```python
from build123d import *
from build123d import SkipClean  # not in build123d's __all__

# Parameters (mm, degrees)
F1_DEPTH     = 2.5
F2_R         = 12
F2_R_2       = 9
F3_DEPTH     = 1.5
F5_DEPTH     = 3
F6_SIZE      = 1.99999
F7_SIZE      = 0.49999
F8_T3_ANGLE  = 65.5786890643
F8_T6_ANGLE  = 65.5786890643
F8_T9_ANGLE  = 65.5786890643
F8_T12_ANGLE = 65.5786890643


# Not quite as in the source:
# - a fillet or chamfer that OpenCascade refuses, or shapes differently, is made with other operations: its cross-section is extruded or revolved along the edge and cut away or added
# - a fillet or chamfer is up to 0.001 mm smaller than in the source, because OpenCascade refuses the exact size


with BuildPart() as f1:
    # F0 (on Front) → F1 (new body)
    with BuildSketch(Plane.XZ):
        with BuildLine():
            Line((-8.0321912081, 4.060037487), (-9.3329510623, 4.811031539))
            ThreePointArc((-9.3329510623, 4.811031539), (-10.5, 0), (-9.3329510623, -4.811031539))
            Line((-9.3329510623, -4.811031539), (-8.0321912081, -4.060037487))
            ThreePointArc((-8.0321912081, -4.060037487), (-9, 0), (-8.0321912081, 4.060037487))
        make_face()
    extrude(amount=-F1_DEPTH)



with BuildPart() as f1b:
    # F0 (on Front) → F1, piece 2 (new body)
    with BuildSketch(Plane.XZ):
        with BuildLine():
            ThreePointArc((8.8329510623, 5.6770569427), (0, 10.5), (-8.8329510623, 5.6770569427))
            Line((-8.8329510623, 5.6770569427), (-7.5321912081, 4.9260628908))
            ThreePointArc((-7.5321912081, 4.9260628908), (0, 9), (7.5321912081, 4.9260628908))
            Line((7.5321912081, 4.9260628908), (8.8329510623, 5.6770569427))
        make_face()
    extrude(amount=-F1_DEPTH)


with BuildPart() as f1c:
    # F0 (on Front) → F1, piece 3 (new body)
    with BuildSketch(Plane.XZ):
        with BuildLine():
            Line((8.0321912081, -4.060037487), (9.3329510623, -4.811031539))
            ThreePointArc((9.3329510623, -4.811031539), (10.5, 0), (9.3329510623, 4.811031539))
            Line((9.3329510623, 4.811031539), (8.0321912081, 4.060037487))
            ThreePointArc((8.0321912081, 4.060037487), (9, 0), (8.0321912081, -4.060037487))
        make_face()
    extrude(amount=-F1_DEPTH)


with BuildPart() as f1d:
    # F0 (on Front) → F1, piece 4 (new body)
    with BuildSketch(Plane.XZ):
        with BuildLine():
            Line((-7.5321912081, -4.9260628908), (-8.8329510623, -5.6770569427))
            ThreePointArc((-8.8329510623, -5.6770569427), (0, -10.5), (8.8329510623, -5.6770569427))
            Line((8.8329510623, -5.6770569427), (7.5321912081, -4.9260628908))
            ThreePointArc((7.5321912081, -4.9260628908), (0, -9), (-7.5321912081, -4.9260628908))
        make_face()
    extrude(amount=-F1_DEPTH)


with BuildPart() as f1_1:
    add(f1.part, clean=False)

    add(f1b.part)  # F3 merges F1b

    add(f1c.part)  # F3 merges F1c

    add(f1d.part)  # F3 merges F1d
    # F2 (on face) → F3 (join)
    with BuildSketch(Plane(origin=(0, 2.5, 0), x_dir=(-1, 0, 0), z_dir=(0, 1, 0))):
        Circle(F2_R)
        Circle(F2_R_2, mode=Mode.SUBTRACT)
    extrude(amount=F3_DEPTH)

    # F4 (on face) → F5 (join)
    with BuildSketch(Plane.XZ):
        with BuildLine():
            ThreePointArc((-7.5321912081, 4.9260628908), (0, 9), (7.5321912081, 4.9260628908))
            Line((7.5321912081, 4.9260628908), (8.8329510623, 5.6770569427))
            ThreePointArc((8.8329510623, 5.6770569427), (0, 10.5), (-8.8329510623, 5.6770569427))
            Line((-8.8329510623, 5.6770569427), (-7.5321912081, 4.9260628908))
        make_face()
        with BuildLine():
            Line((8.0321912081, -4.060037487), (9.7664331553, -5.0613025421))
            ThreePointArc((9.7664331553, -5.0613025421), (11, 0), (9.7664331553, 5.0613025421))
            Line((9.7664331553, 5.0613025421), (8.0321912081, 4.060037487))
            ThreePointArc((8.0321912081, 4.060037487), (9, 0), (8.0321912081, -4.060037487))
        make_face()
        with BuildLine():
            Line((-8.0321912081, 4.060037487), (-9.7664331553, 5.0613025421))
            ThreePointArc((-9.7664331553, 5.0613025421), (-11, 0), (-9.7664331553, -5.0613025421))
            Line((-9.7664331553, -5.0613025421), (-8.0321912081, -4.060037487))
            ThreePointArc((-8.0321912081, -4.060037487), (-9, 0), (-8.0321912081, 4.060037487))
        make_face()
        with BuildLine():
            Line((-7.5321912081, -4.9260628908), (-8.8329510623, -5.6770569427))
            ThreePointArc((-8.8329510623, -5.6770569427), (0, -10.5), (8.8329510623, -5.6770569427))
            Line((8.8329510623, -5.6770569427), (7.5321912081, -4.9260628908))
            ThreePointArc((7.5321912081, -4.9260628908), (0, -9), (-7.5321912081, -4.9260628908))
        make_face()
    with SkipClean():  # cleaning this boolean's faces spoils the solid; the shape is the same uncleaned
        extrude(amount=F5_DEPTH)

    # F6 (size 2 in the source; OpenCascade refuses exactly that, so slightly less here)
    f6_edges = [f1_1.edges().sort_by_distance(p)[0] for p in [
        (-11, -3, 0),
        (11, -3, 0),
    ]]
    chamfer(f6_edges, length=F6_SIZE)

    # F7 (size 0.5 in the source; OpenCascade refuses exactly that, so slightly less here)
    f7_edges = [f1_1.edges().sort_by_distance(p)[0] for p in [
        (-11, 0, 0),
        (11, 0, 0),
    ]]
    chamfer(f7_edges, length=F7_SIZE)

    # F8: fillet of radius 1 on 4 edges, made by hand


with BuildPart() as f8_tool1:
    # F8_s2 → F8_t3 (revolve)
    with BuildSketch(Plane(origin=(0, 0, 0), x_dir=(0, 1, 0), z_dir=(0.5415518782, 0, 0.8406673321))):
        with BuildLine():
            ThreePointArc((-0.5857964376, 11), (-0.96847987, 10.9238795325), (-1.2929032188, 10.7071067812))
            Line((-1.2929032188, 10.7071067812), (-1.00001, 11))
            Line((-1.00001, 11), (-0.5857964376, 11))
        make_face()
    revolve(axis=Axis((0, -1.00001, 0), (0, -1, 0)), revolution_arc=F8_T3_ANGLE)


with BuildPart() as f8_tool4:
    # F8_s5 → F8_t6 (revolve)
    with BuildSketch(Plane(origin=(0, 0, 0), x_dir=(0, 1, 0), z_dir=(0.5415518782, 0, 0.8406673321))):
        with BuildLine():
            ThreePointArc((-0.9142035624, 11), (-0.53152013, 10.9238795325), (-0.2070967812, 10.7071067812))
            Line((-0.2070967812, 10.7071067812), (-0.49999, 11))
            Line((-0.49999, 11), (-0.9142035624, 11))
        make_face()
    revolve(axis=Axis((0, -0.49999, 0), (0, -1, 0)), revolution_arc=F8_T6_ANGLE)


with BuildPart() as f8_tool7:
    # F8_s8 → F8_t9 (revolve)
    with BuildSketch(Plane(origin=(0, 0, 0), x_dir=(0, 1, 0), z_dir=(-0.5415518782, 0, -0.8406673321))):
        with BuildLine():
            ThreePointArc((-0.5857964376, 11), (-0.96847987, 10.9238795325), (-1.2929032188, 10.7071067812))
            Line((-1.2929032188, 10.7071067812), (-1.00001, 11))
            Line((-1.00001, 11), (-0.5857964376, 11))
        make_face()
    revolve(axis=Axis((0, -1.00001, 0), (0, -1, 0)), revolution_arc=F8_T9_ANGLE)


with BuildPart() as f8_tool10:
    # F8_s11 → F8_t12 (revolve)
    with BuildSketch(Plane(origin=(0, 0, 0), x_dir=(0, 1, 0), z_dir=(-0.5415518782, 0, -0.8406673321))):
        with BuildLine():
            ThreePointArc((-0.9142035624, 11), (-0.53152013, 10.9238795325), (-0.2070967812, 10.7071067812))
            Line((-0.2070967812, 10.7071067812), (-0.49999, 11))
            Line((-0.49999, 11), (-0.9142035624, 11))
        make_face()
    revolve(axis=Axis((0, -0.49999, 0), (0, -1, 0)), revolution_arc=F8_T12_ANGLE)


with BuildPart() as f1_2:
    add(f1_1.part, clean=False)

    # F8_t13: cut F8_tool1, F8_tool4, F8_tool7, F8_tool10
    add([f8_tool1.part, f8_tool4.part, f8_tool7.part, f8_tool10.part], mode=Mode.SUBTRACT)


solid = f1_2.part
```
Geometry check sheet. Reference: the model listing, model coordinates, mm. A direction names the side the tool comes from. Give positions to 0.01 mm unless a question says otherwise; leave off trailing zeros. Write each loop counter-clockwise with the first axis right and the second up, starting at its lowest first coordinate (ties: lowest second). Pieces come first, ordered by that corner, then holes. Notation, with made-up numbers: (77, -0.5) - (106, -0.5) arc R19 cw to (106, 6.5) - close; hole circle Ø9 at (-32, 66). An arc over 180 degrees is marked (long way). Use a Markdown table: item, result.
Q1. Section check B-B, the plane z = -7.25. Enter the section's corners in (x, y).
Computed:
| item | result |
|---|---|
| outline | (-9.56, 2.5) - (-7.6, 2.5) - (-7.6, -3) - (-5.33, -3) - (-5.33, 4) - (-9.56, 4) - close; (5.33, -3) - (7.6, -3) - (7.6, 2.5) - (9.56, 2.5) - (9.56, 4) - (5.33, 4) - close |
Q2. Thickness scan on L1, parallel to Z at x = 0, y = 0; L2, parallel to X at y = 2.75, z = 3.75; L3, parallel to Y at x = 7, z = -9.5. Record the ranges inside material, lowest first. Write a range as [from, to].
Computed:
| item | result |
|---|---|
| L1 | z = [-10.5, -9], [9, 10.5] |
| L2 | x = [-11.4, -8.18], [8.18, 11.4] |
| L3 | y = [2.5, 4] |
Q3. Draft check along Z on faces 4 (the face through (11.99, 3.24, 0.53)), 5 (the face through (0.1, -0.3, 10.5)), 6 (the face through (-8.173, -0.288, -5.296)). Enter one of: pulls with the +Z half, pulls with the -Z half, needs draft (parallel to the pull), parting line crosses it, or undercut.
Computed:
| item | result |
|---|---|
| face 4 | parting line crosses it |
| face 5 | pulls with the +Z half |
| face 6 | undercut |
Q4. Section check A-A, the plane y = 1.5. Enter the section's corners in (x, z).
Computed:
| item | result |
|---|---|
| outline | (-9.33, -4.81) - (-8.03, -4.06) arc R9 cw to (-8.03, 4.06) - (-9.33, 4.81) arc R10.5 ccw to start; (-8.83, -5.68) arc R10.5 ccw to (8.83, -5.68) - (7.53, -4.93) arc R9 cw to (-7.53, -4.93) - close; (-8.83, 5.68) - (-7.53, 4.93) arc R9 cw to (7.53, 4.93) - (8.83, 5.68) arc R10.5 ccw to start; (8.03, -4.06) - (9.33, -4.81) arc R10.5 ccw to (9.33, 4.81) - (8.03, 4.06) arc R9 cw to start |
Q5. Section check D-D, the plane y = -2. Enter the section's corners in (x, z).
Computed:
| item | result |
|---|---|
| outline | (-8.9, -4.56) - (-8.03, -4.06) arc R9 cw to (-8.03, 4.06) - (-8.9, 4.56) arc R10 ccw to start; (-8.83, -5.68) arc R10.5 ccw to (8.83, -5.68) - (7.53, -4.93) arc R9 cw to (-7.53, -4.93) - close; (-8.83, 5.68) - (-7.53, 4.93) arc R9 cw to (7.53, 4.93) - (8.83, 5.68) arc R10.5 ccw to start; (8.03, -4.06) - (8.9, -4.56) arc R10 ccw to (8.9, 4.56) - (8.03, 4.06) arc R9 cw to start |
Q6. Go/stop test with flat-tipped pins: P1, Ø4, axis at y = 1.5, z = 8, coming from the +X side; P2, Ø3, axis at x = -6.5, z = 5.5, coming from the +Y side; P3, Ø1.5, axis at x = -3, y = 2.5, coming from the +Z side. Record where each tip stops, or that it passes through.
Computed:
| item | result |
|---|---|
| P1 | stops at x = 10.23 |
| P2 | stops at y = 4 |
| P3 | stops at z = 11.79 |
Q7. Set-up check for faces 1 (the face through (-0.1, -0.3, -10.5)), 2 (the face through (10.5, 1.2, -0.1)), 3 (the face through (-10.5, 1.2, 0.1)): record each of +Z, -Z, +X, -X, +Y, -Y from which the full face is reachable in a straight line by a thin tool's end or side.
Computed:
| item | result |
|---|---|
| face 1 | -Z, -Y |
| face 2 | +X |
| face 3 | -X |
Q8. Section check C-C, the plane x = 0. Enter the section's corners in (y, z), then the cut area to 3 significant figures.
Computed:
| item | result |
|---|---|
| outline | (-3, -10.5) - (2.5, -10.5) - (2.5, -12) - (4, -12) - (4, -9) - (-3, -9) - close; (-3, 9) - (4, 9) - (4, 12) - (2.5, 12) - (2.5, 10.5) - (-3, 10.5) - close |
| area | 25.5 mm² |
